Could you check a few things on this model? Use its own coordinates, in mm. Face numbers are marked on the shaded views. A direction names the side the tool comes from. Coordinates: 2 decimals unless noted, no trailing zeros. Loops run counter-clockwise (first coordinate to the right, second up) from the corner with the lowest first, then second, coordinate; pieces in that order, holes last.
1) Imagine slicing it at C-C on x = -1. Give the number of separate pieces and of enclosed holes in the cut face, plus the area to 3 significant figures.
2) If I drill on line 1 along Y through (x, z) = (4.7, -11.36); line 2 along Y through (x, z) = (-4.25, -23); line 3 along Z through (x, y) = (0.75, 15.25), over which ranges is the centre line in solid material (lowest first)?
3) Imagine slicing it at B-B on y = -3.5. Please give me the cut outline in (x, z).
4) Will these pins go through, and if not, where does the flat tip stop? P1, Ø2, axis at x = -3.5, z = -14.5, coming from the +Y side; P2, Ø3, axis at x = -2, y = 9, coming from the +Z side; P3, Ø5, axis at y = -3.5, z = -11.36, coming from the -X side.
5) For the marked faces 4, 5, 6, 7 and 8, which set-ups out of +Z, -Z, +X, -X, +Y, -Y let a thin tool reach every point of the face, with its end or its side?
6) Imagine slicing it at A-A on z = -21.36. Please give me the cut outline in (x, y), plus the area to 3 significant figures.
7) Thinking about a two-plate mould opening in Z: for the marked faces 1, 2 and 3, which applies, released by +Z, released by -Z, zero draft, split by the parting line, or undercut?
```python
from build123d import *

# Parameters (mm, degrees)
CROQUIS1_R              = 1.5
SALIENTE_EXTRUIR1_DEPTH = 2.5
SALIENTE_EXTRUIR2_START = 8.15
CROQUIS1_3_R            = 2.5
SALIENTE_EXTRUIR2_DEPTH = 7.87
SALIENTE_EXTRUIR5_DEPTH = 16.02
REDONDEO3_R             = 5
CROQUIS8_W              = 22.36
CROQUIS8_H              = 7.5
CROQUIS8_R              = 1.5
SALIENTE_EXTRUIR6_DEPTH = 2.5


with BuildPart() as part:
    # Croquis1 → Saliente-Extruir1 (new body)
    with BuildSketch(Plane(origin=(0, 0, 0), x_dir=(1, 0, 0), z_dir=(0, 1, 0))):
        Polygon((3.6, 27.36), (-7.02, 27.36), (-5.314994069, 13.6091097), (3.6, 5), align=None)
        with Locations(Location((-0.4, 21.36, 0), (0, 0, 270))):
            Circle(CROQUIS1_R, mode=Mode.SUBTRACT)
    extrude(amount=SALIENTE_EXTRUIR1_DEPTH)



with BuildPart() as body_2:
    # Croquis1<3> → Saliente-Extruir2 (new body)
    with BuildSketch(Plane(origin=(0, 0, 0), x_dir=(1, 0, 0), z_dir=(0, 1, 0)).offset(SALIENTE_EXTRUIR2_START)):
        with BuildLine():
            Line((3.6, 5), (-5.314994069, 13.6091097))
            Line((-5.314994069, 13.6091097), (-3.572641648, -0.442980423))
            ThreePointArc((-3.572641648, -0.442980423), (0.221912221, -3.593153902), (3.6, 0))
            Line((3.6, 0), (3.6, 5))
        make_face()
        with Locations(Location((0, 0, 0), (0, 0, 270))):
            Circle(CROQUIS1_3_R, mode=Mode.SUBTRACT)
    extrude(amount=SALIENTE_EXTRUIR2_DEPTH)


with BuildPart() as part_1:
    add(part.part)

    add(body_2.part)  # Saliente-Extruir5 merges body 2
    # Croquis1<6> → Saliente-Extruir5 (add)
    with BuildSketch(Plane(origin=(0, 0, 0), x_dir=(1, 0, 0), z_dir=(0, 1, 0))):
        Polygon((3.6, 11.25573616), (-6.196167881, 20.715785518), (-5.314994069, 13.6091097), (3.6, 5), align=None)
    extrude(amount=SALIENTE_EXTRUIR5_DEPTH)

    # Redondeo3
    redondeo3_edges = [part_1.edges().sort_by_distance(p)[0] for p in [
        (-1.29808394, 16.02, -15.985760839),
    ]]
    fillet(redondeo3_edges, radius=REDONDEO3_R)

    # Croquis8 → Saliente-Extruir6 (add)
    # profile 1 of 2: a face of its own
    with BuildSketch(Plane(origin=(3.6, 0, 0), x_dir=(0, 0, -1), z_dir=(1, 0, 0))):
        with BuildLine():
            Line((5, 15.994937186), (5, 8.15))
            Line((5, 8.15), (5, 0))
            Line((5, 0), (27.36, 0))
            Line((27.36, 0), (27.36, 2.5))
            Line((27.36, 2.5), (11.25573616, 2.5))
            Line((11.25573616, 2.5), (11.25573616, 11.02))
            add(Edge.make_bspline(
                [(11.25573616, 11.02), (11.25573616, 15.542670169), (5, 15.994937186)],
                knots=[3.141592654, 3.141592654, 3.141592654, 4.603302756, 4.603302756, 4.603302756], degree=2, weights=[1, 0.727447175, 0.962144349]))
        make_face()
    # profile 2 of 2: a face of its own
    with BuildSketch(Plane(origin=(3.6, 0, 0), x_dir=(0, 0, -1), z_dir=(1, 0, 0))):
        with Locations((16.18, -3.75)):
            Rectangle(CROQUIS8_W, CROQUIS8_H)
        with Locations((11.36, -3.5)):
            Circle(CROQUIS8_R, mode=Mode.SUBTRACT)
    extrude(amount=SALIENTE_EXTRUIR6_DEPTH)


solid = part_1.part
```
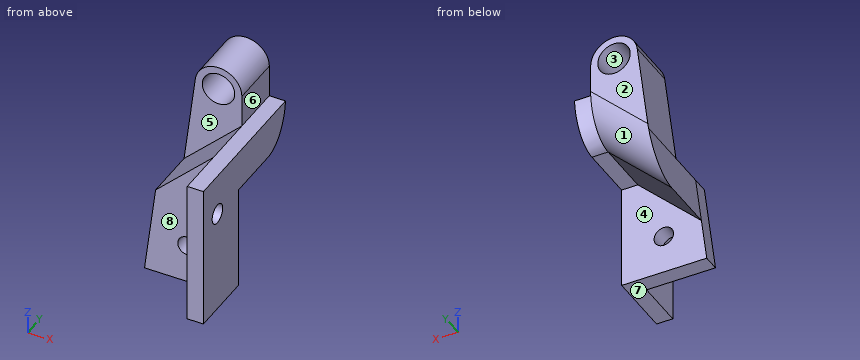
Filled in:
1. separate pieces: 3
1. enclosed holes: 0
1. area: 181 mm2
2. line 1: y = -7.5 to -5, -2 to 2.5
2. line 2: y = 0 to 2.5
2. line 3: z = -10.76 to -2.38, 2.38 to 3.52
3. outline: (3.6, -27.36) - (6.1, -27.36) - (6.1, -12.86) - (3.6, -12.86) - close; (3.6, -9.86) - (6.1, -9.86) - (6.1, -5) - (3.6, -5) - close
4. P1: stops at y = 15.82
4. P2: stops at z = 3.57
4. P3: stops at x = 3.6
5. face 4: -Z, +X, +Y
5. face 5: +Z, -X, -Y
5. face 6: +Z, +X, +Y, -Y
5. face 7: -Z, +X, -X, +Y, -Y
5. face 8: +Z, -Z, -X, -Y
6. outline: (-6.28, 0) - (-1.9, 0) - (-1.9, 2.5) - (-6.28, 2.5) - close; (1.1, 0) - (3.6, 0) - (3.6, -7.5) - (6.1, -7.5) - (6.1, 2.5) - (1.1, 2.5) - close
6. area: 42.2 mm2
7. face 1: released by -Z
7. face 2: zero draft
7. face 3: undercut
